The model under review builds one solid part; all positions refer to its coordinate system, in mm. A direction names the side the tool comes from. Round coordinates to 2 decimals unless told otherwise and drop trailing zeros. Write each loop counter-clockwise with the first axis right and the second up, starting at its lowest first coordinate (ties: lowest second). Pieces come first, ordered by that corner, then holes. Notation, with made-up numbers: (14, 85.25) - (55, 85.25) arc R30 ccw to (55, 109.25) - close; hole circle Ø7 at (82, 80.25). An arc over 180 degrees is marked (long way). Return JSON: item names as keys, results as strings.
from build123d import *

# Parameters (mm, degrees)
F1_DEPTH = 20
F2_R     = 1
F4_D     = 3.2
F5_SIZE  = 0.5


with BuildPart() as f1:
    # F0 (on Front) → F1 (new body)
    with BuildSketch(Plane.XZ):
        Polygon((-10.72, 30.72), (-5, 30.72), (-2.5, 28.22), (2.5, 28.22), (5, 30.72), (5, 32.72), (-12.72, 32.72), (-12.72, -32.72), (5, -32.72), (5, -30.72), (2.5, -28.22), (-2.5, -28.22), (-5, -30.72), (-10.72, -30.72), (-10.72, -25), (-8.22, -22.5), (-8.22, -17.5), (-10.72, -15), (-10.72, -5), (-8.22, -2.5), (-8.22, 2.5), (-10.72, 5), (-10.72, 15), (-8.22, 17.5), (-8.22, 22.5), (-10.72, 25), align=None)
    extrude(amount=F1_DEPTH)

    # F2
    f2_edges = [f1.edges().sort_by_distance(p)[0] for p in [
        (5, -10, 32.72),
        (-12.72, -10, 32.72),
        (-12.72, -10, -32.72),
        (5, -10, -32.72),
    ]]
    fillet(f2_edges, radius=F2_R)

    # F4 (through all)
    with Locations(Plane(origin=(-12.72, 0, 0), x_dir=(0, -1, 0), z_dir=(-1, 0, 0))):
        with Locations((10, 20), (10, 0), (10, -20)):
            Hole(F4_D / 2)

    # F5
    f5_edges = [f1.edges().sort_by_distance(p)[0] for p in [
        (5, -20, 31.22),
        (4.707107, -20, 32.427107),
        (3.75, -20, 29.47),
        (-3.86, -20, 32.72),
        (0, -20, 28.22),
        (-12.427107, -20, 32.427107),
        (-3.75, -20, 29.47),
        (-12.72, -20, 0),
        (-7.86, -20, 30.72),
        (-12.427107, -20, -32.427107),
        (-10.72, -20, 27.86),
        (-3.86, -20, -32.72),
        (-9.47, -20, 23.75),
        (4.707107, -20, -32.427107),
        (-8.22, -20, 20),
        (5, -20, -31.22),
        (-9.47, -20, 16.25),
        (3.75, -20, -29.47),
        (-10.72, -20, 10),
        (0, -20, -28.22),
        (-9.47, -20, 3.75),
        (-3.75, -20, -29.47),
        (-8.22, -20, 0),
        (-7.86, -20, -30.72),
        (-9.47, -20, -3.75),
        (-10.72, -20, -27.86),
        (-10.72, -20, -10),
        (-9.47, -20, -23.75),
        (-9.47, -20, -16.25),
        (-8.22, -20, -20),
        (5, 0, 31.22),
        (4.707107, 0, 32.427107),
        (3.75, 0, 29.47),
        (-3.86, 0, 32.72),
        (0, 0, 28.22),
        (-12.427107, 0, 32.427107),
        (-3.75, 0, 29.47),
        (-12.72, 0, 0),
        (-7.86, 0, 30.72),
        (-12.427107, 0, -32.427107),
        (-10.72, 0, 27.86),
        (-3.86, 0, -32.72),
        (-9.47, 0, 23.75),
        (4.707107, 0, -32.427107),
        (-8.22, 0, 20),
        (5, 0, -31.22),
        (-9.47, 0, 16.25),
        (3.75, 0, -29.47),
        (-10.72, 0, 10),
        (0, 0, -28.22),
        (-9.47, 0, 3.75),
        (-3.75, 0, -29.47),
        (-8.22, 0, 0),
        (-7.86, 0, -30.72),
        (-9.47, 0, -3.75),
        (-10.72, 0, -27.86),
        (-10.72, 0, -10),
        (-9.47, 0, -23.75),
        (-9.47, 0, -16.25),
        (-8.22, 0, -20),
    ]]
    chamfer(f5_edges, length=F5_SIZE)


solid = f1.part
(1) Wall thickness on line 1 (Z direction, x = -11, y = -10); line 2 (Z direction, x = -1, y = -9); line 3 (X direction, y = -18.5, z = 12): over which ranges is each line inside the solid? List them lowest first.
Filled in:
{"line 1": "z = -32.72 to -21.6, -18.4 to -1.6, 1.6 to 18.4, 21.6 to 32.72", "line 2": "z = -32.72 to -28.22, 28.22 to 32.72", "line 3": "x = -12.72 to -10.72"}
(2) Clearance check with flat-ended pins moving along their axes: pin 1 Ø8 at (y, z) = (-14.5, -10) entering from +X; pin 2 Ø3 at (x, z) = (1, 25.5) entering from -Y; pin 3 Ø1.5 at (y, z) = (-7, 19) entering from +X; pin 4 Ø4.5 at (y, z) = (-8.5, 27.5) entering from +X. State where each tip first meets the part, or that it passes through.
Filled in:
{"pin 1": "stops at x = -10.72", "pin 2": "passes through", "pin 3": "stops at x = -8.22", "pin 4": "stops at x = 4.03"}
(3) Add section B-B (x = -6.75). Write out the cut boundary in (y, z), plus the area to 3 significant figures.
Filled in:
{"outline": "(-20, -32.22) - (-19.5, -32.72) - (-0.5, -32.72) - (0, -32.22) - (0, -31.22) - (-0.5, -30.72) - (-19.5, -30.72) - (-20, -31.22) - close; (-20, 31.22) - (-19.5, 30.72) - (-0.5, 30.72) - (0, 31.22) - (0, 32.22) - (-0.5, 32.72) - (-19.5, 32.72) - (-20, 32.22) - close", "area": "79.0 mm2"}
(4) Mouldability with a two-part tool opening along Z and no side actions: class faces 1 (the flat face through (-12.72, -8, 0)), 2 (the flat face through (3.73, -9.87, 29.45)), 3 (the flat face through (-4, -10, -32.72)) as released by +Z, released by -Z, zero draft, split by the parting line, or undercut.
Filled in:
{"face 1": "zero draft", "face 2": "undercut", "face 3": "released by -Z"}
(5) Add section D-D (y = -10). Give the number of separate pieces and of enclosed holes in the cut face, plus the area to 3 significant figures.
Filled in:
{"separate pieces": "4", "enclosed holes": "0", "area": "243 mm2"}
(6) For faces 4 (the flat face through (-3.73, -9.87, -29.45)), 5 (the flat face through (-3.7, -19.7, 29.7)), 6 (the flat face through (3.59, -0.25, -29.66)), list the 3-axis set-ups (+Z, -Z, +X, -X, +Y, -Y) from which the entire face can be reached by the end or side of a thin tool; tool diameter is ignored.
Filled in:
{"face 4": "+Y, -Y", "face 5": "-Y", "face 6": "+X, +Y"}
(7) Add section A-A (z = 20). Write out the cut boundary in (x, y).
Filled in:
{"outline": "(-12.72, -19.5) - (-12.22, -20) - (-8.72, -20) - (-8.22, -19.5) - (-8.22, -11.6) - (-12.72, -11.6) - close; (-12.72, -8.4) - (-8.22, -8.4) - (-8.22, -0.5) - (-8.72, 0) - (-12.22, 0) - (-12.72, -0.5) - close"}
